Verification items for the finished model (mm, model axes). Give positions to 0.01 mm unless a question says otherwise; leave off trailing zeros. Order: outer loops, then holes, each group sorted by start corner. A loop starts at its lowest first (then second) coordinate and runs counter-clockwise, first axis right, second up. Notation, with made-up numbers: (43, -35.5) -> (95, -35.5) arc R22 cw to (95, -2.5) -> close; hole circle Ø1 at (-37.5, 64.25). An arc over 180 degrees is marked (long way). Return JSON: item names as keys, results as strings. Group by question number.
(1) Depth check by flat-ended pin: pin 1 Ø5 at (x, y) = (64, 12) entering from +Z. Enter the tip coordinate at first touch or a pass-through.
(2) Thickness scan on line 1 along Y through (x, z) = (-64.25, 2.4); line 2 along X through (y, z) = (-12, 1.1); line 3 along Y through (x, z) = (64.25, 0.9). Record the ranges inside material, lowest first.
(3) Cross-section at A-A on x = -64.25. Enter the section's corners in (y, z).
(4) Cross-section at B-B on y = -12. State how many separate pieces and enclosed holes the cut face has, then the cut area to 3 significant figures.
Autodesk Inventor part; units mm, degrees
ref_plane "YZ Plane" through (0, 0, 0) normal (1, 0, 0) x (0, 1, 0)
ref_plane "XZ Plane" through (0, 0, 0) normal (0, 1, 0) x (-1, 0, 0)
ref_plane "XY Plane" through (0, 0, 0) normal (0, 0, 1) x (1, 0, 0)
sketch "Sketch1" plane through (0, 0, 0) normal (0, 0, 1) x (1, 0, 0)
  line L0 (-71, -15.75) -> (71, -15.75)
  line L1 (72, -14.75) -> (72, 14.75)
  line L2 (71, 15.75) -> (-71, 15.75)
  line L3 (-72, 14.75) -> (-72, -14.75)
  line L4 (-72, -15.75) -> (72, 15.75) construction
  line L5 (72, -15.75) -> (-72, 15.75) construction
  line L6 (0, 0) -> (0, 12) construction
  line L7 (0, 12) -> (64.25, 12) construction
  line L8 (0, 12) -> (-64.25, 12) construction
  line L9 (0, 0) -> (34.0768, 0) construction
  circle A0 centre (-64.25, 12) radius 1.75
  circle A1 centre (0, 12) radius 1.75
  circle A2 centre (64.25, 12) radius 1.75
  circle A3 centre (-64.25, -12) radius 1.75
  circle A4 centre (0, -12) radius 1.75
  circle A5 centre (64.25, -12) radius 1.75
  arc A6 (-71, 15.75) -> (-72, 14.75) centre (-71, 14.75) ccw
  arc A7 (72, 14.75) -> (71, 15.75) centre (71, 14.75) ccw
  arc A8 (71, -15.75) -> (72, -14.75) centre (71, -14.75) ccw
  arc A9 (-72, -14.75) -> (-71, -15.75) centre (-71, -14.75) ccw
  dimension "d0" = 144
  dimension "d1" = 31.5
  dimension "d2" = 64.25
  dimension "d3" = 12
  dimension "d4" = 3.5
  dimension "d5" = 1
extrude "Extrusion1" add sketch "Sketch1" along normal blind 4
sketch "Sketch2" plane through (0, 0, 4) normal (0, 0, 1) x (1, 0, 0)
  circle A0 centre (-64.25, 12) radius 1.75
  circle A1 centre (-64.25, 12) radius 3
  circle A2 centre (0, 12) radius 1.75
  circle A3 centre (0, 12) radius 3
  circle A4 centre (64.25, 12) radius 1.75
  circle A5 centre (64.25, 12) radius 3
  circle A6 centre (64.25, -12) radius 1.75
  circle A7 centre (64.25, -12) radius 3
  circle A8 centre (0, -12) radius 1.75
  circle A9 centre (0, -12) radius 3
  circle A10 centre (-64.25, -12) radius 1.75
  circle A11 centre (-64.25, -12) radius 3
  point P0 (0, 0)
  dimension "d8" = 6
extrude "Extrusion2" cut sketch "Sketch2" against normal blind 2.2 contours A0 | A1 | A2 | A3 | A4 | A5 | A6 | A7 | A8 | A9 | A10 | A11
fillet "Fillet1" radius 0.5 16 edges at (-71.7071, 15.4571, 4) (-72, 0, 4) (-71.7071, -15.4571, 4) (0, -15.75, 4) (71.7071, -15.4571, 4) (72, 0, 4) (71.7071, 15.4571, 4) (0, 15.75, 4) (71.7071, -15.4571, 0) (72, 0, 0) (71.7071, 15.4571, 0) (0, 15.75, 0) (-71.7071, 15.4571, 0) (-72, 0, 0) (-71.7071, -15.4571, 0) (0, -15.75, 0)
properties part number "Link2_FlatCover"
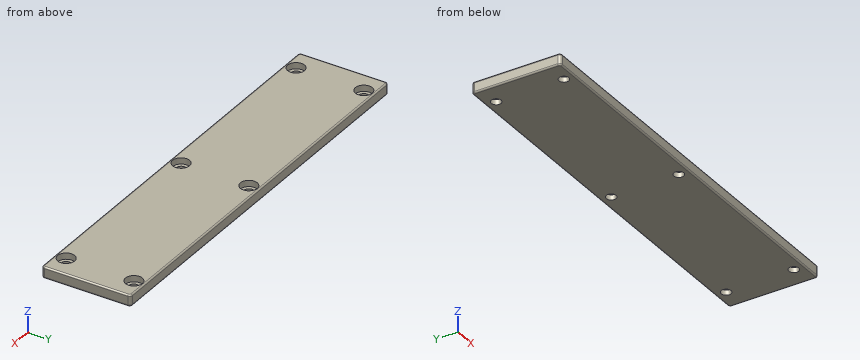
Verdict:
{
 "1": {"pin 1": "z = 1.8"},
 "2": {"line 1": "-15.75 to -15, -9 to 9, 15 to 15.75", "line 2": "-72 to -66, -62.5 to -1.75, 1.75 to 62.5, 66 to 72", "line 3": "-15.75 to -13.75, -10.25 to 10.25, 13.75 to 15.75"},
 "3": {"outline": "(-15.75, 0.5) arc R0.5 ccw to (-15.25, 0) -> (-13.75, 0) -> (-13.75, 1.8) -> (-15, 1.8) -> (-15, 4) -> (-15.25, 4) arc R0.5 ccw to (-15.75, 3.5) -> close; (-10.25, 0) -> (10.25, 0) -> (10.25, 1.8) -> (9, 1.8) -> (9, 4) -> (-9, 4) -> (-9, 1.8) -> (-10.25, 1.8) -> close; (13.75, 0) -> (15.25, 0) arc R0.5 ccw to (15.75, 0.5) -> (15.75, 3.5) arc R0.5 ccw to (15.25, 4) -> (15, 4) -> (15, 1.8) -> (13.75, 1.8) -> close"},
 "4": {"separate pieces": "4", "enclosed holes": "0", "area": "517 mm²"}
}
